For this review, take the finished solid that the model builds, in its own axes (mm). A direction names the side the tool comes from. Coordinates: 2 decimals unless noted, no trailing zeros. Order: outer loops, then holes, each group sorted by start corner. A loop starts at its lowest first (then second) coordinate and runs counter-clockwise, first axis right, second up. Notation, with made-up numbers: M 63.5,84.5 L 93.5,84.5 A25 ccw 93.5,103.5 Z; hole C 70,2.25 d2. An arc over 180 degrees is marked long. Use CSV: the item, a comma, the result in double quotes.
```python
from build123d import *

# Parameters (mm, degrees)
F1_DEPTH  = 41.275
F2_R      = 9.525
F3_DEPTH  = 53.34
F5_W      = 260.929487
F5_H      = 28.83905
F6_DEPTH  = 22.1996
F8_DEPTH  = 50.8
F9_R      = 1.2954
F10_DEPTH = 101.6
F11_R     = 1.2954
F12_DEPTH = 101.6


with BuildPart() as f1:
    # F0 (on Front) → F1 (new body)
    with BuildSketch(Plane.XZ):
        Polygon((-73.813496, 63.5), (-73.813496, 0), (222.924162, 0), (222.924162, 20.32), align=None)
    extrude(amount=-F1_DEPTH)

    # F2 (on face) → F3 (cut)
    with BuildSketch(Plane(origin=(-73.813496, 0, 0), x_dir=(0, -1, 0), z_dir=(-1, 0, 0))):
        with Locations((-20.6375, 31.75)):
            Circle(F2_R)
    extrude(amount=-F3_DEPTH, mode=Mode.SUBTRACT)

    # F5 (on face) → F6 (cut)
    with BuildSketch(Plane(origin=(0, 0, 0), x_dir=(1, 0, 0), z_dir=(0, 0, -1))):
        with Locations((70.18033, -21.463492)):
            Rectangle(F5_W, F5_H)
    extrude(amount=-F6_DEPTH, mode=Mode.SUBTRACT)

    # F7 (on face) → F8 (cut)
    with BuildSketch(Plane.XZ):
        Polygon((-24.655161, 45.214526), (167.490213, 28.386512), (-73.813496, 63.5), (-73.813496, 53.013064), (-51.996879, 53.013064), align=None)
    extrude(amount=-F8_DEPTH, mode=Mode.SUBTRACT)

    # F9 (on face) → F10 (cut)
    with BuildSketch(Plane.XZ):
        with Locations((0, 8.893992)):
            Circle(F9_R)
    extrude(amount=-F10_DEPTH, mode=Mode.SUBTRACT)

    # F11 (on face) → F12 (cut)
    with BuildSketch(Plane.XZ):
        with Locations((153.94105, 8.016577)):
            Circle(F11_R)
    extrude(amount=-F12_DEPTH, mode=Mode.SUBTRACT)


solid = f1.part
```
Item 1: Add section B-B on z = 38. State the section outline as (x, y) points (1 decimal), and give its area (3 significant figures).
Solutions:
outline,"M -73.8,0 L 57.7,0 L 57.7,41.3 L -73.8,41.3 L -73.8,27.8 L -20.5,27.8 L -20.5,13.4 L -73.8,13.4 Z"
area,"4,660 mm^2"
Item 2: Draft analysis for pull direction Y (two halves, no side actions). For faces 4 (the face through (-47.52, 22.7, 22.45)), 5 (the face through (40, 0, 21)), 6 (the face through (-63, 20, 53.013)), state which applies: released by +Y, released by -Y, zero draft, split by the parting line, or undercut.
Solutions:
face 4,"undercut"
face 5,"released by -Y"
face 6,"zero draft"
Item 3: Add section C-C on x = 104. State the section outline as (y, z) points (3 decimals).
Solutions:
outline,"M 0,0 L 7.044,0 L 7.044,22.2 L 35.883,22.2 L 35.883,0 L 41.275,0 L 41.275,33.947 L 0,33.947 Z"
Item 4: Clearance check with flat-ended pins moving along their axes: pin 1 Ø8.5 at (x, y) = (39.5, 28.5) entering from -Z; pin 2 Ø5 at (x, y) = (169, 7.5) entering from +Z; pin 3 Ø1 at (x, y) = (169, 28) entering from +Z; pin 4 Ø1.6 at (x, z) = (153.94, 8.02) entering from +Y. State where each tip first meets the part, or that it passes through.
Solutions:
pin 1,"z = 22.2"
pin 2,"z = 28.47"
pin 3,"z = 28.24"
pin 4,"through"
Item 5: To check wall thickness, follow line 1 along Y through (x, z) = (-47.5, 31) (3 decimals); line 2 along Y through (x, z) = (22, 5) (3 decimals); line 3 along X through (y, z) = (29, 19). State the ranges of each line that lie inside material, in increasing order. Write a range as [from, to].
Solutions:
line 1,"[0, 11.142], [30.133, 41.275]"
line 2,"[0, 7.044], [35.883, 41.275]"
line 3,"[-73.81, -60.28], [200.65, 222.92]"
Item 6: For faces 1 (the face through (-60.284, 22, 11)), 2 (the face through (195.595, 20.349, 24.297)), 3 (the face through (-20.473, 21, 32)), list the 3-axis set-ups (+Z, -Z, +X, -X, +Y, -Y) from which the entire face can be reached by the end or side of a thin tool; tool diameter is ignored.
Solutions:
face 1,"-Z"
face 2,"+Z, +X, +Y, -Y"
face 3,"-X"
Item 7: Add section D-D on y = 20.5. State the section outline as (x, z) points.
Solutions:
outline,"M -73.81,0 L -60.28,0 L -60.28,22.2 L 200.65,22.2 L 200.65,0 L 222.92,0 L 222.92,20.32 L 167.49,28.39 L -24.66,45.21 L -52,53.01 L -73.81,53.01 L -73.81,41.27 L -20.47,41.27 L -20.47,22.23 L -73.81,22.23 Z"
